Can you work these out from the model? Positions are in its coordinate system, mm. Coordinates: 2 decimals unless noted, no trailing zeros. Order: outer loops, then holes, each group sorted by start corner. A loop starts at its lowest first (then second) coordinate and runs counter-clockwise, first axis right, second up. Notation, with made-up numbers: (-32, -7.5) -> (-6, -7.5) arc R17 cw to (-6, 19.5) -> close; hole circle Ø5 at (64.5, -28). An arc over 180 degrees is marked (long way). Answer in a Markdown table with one row per item. Add a question column.
1. If I drill on line 1 along Z through (x, y) = (0, 12.95); line 2 along Y through (x, z) = (1, 5.5); line 3 along Z through (x, y) = (12.5, -8), over which ranges is the centre line in solid material (lowest first)? Write a range as [from, to].
2. Imagine slicing it at A-A on z = 31.5. Write out the boundary of the cut face in (x, y), plus the area to 3 significant figures.
3. Imagine slicing it at B-B on y = 0. Write out the boundary of the cut face in (x, z).
4. Imagine slicing it at C-C on x = -6. Write out the boundary of the cut face in (y, z), plus the area to 3 significant figures.
5. Will these pins go through, and if not, where does the flat tip stop? pin 1 (0.9 mm diameter, centred on y = 14, z = 34, fed in from -X); pin 2 (2 mm diameter, centred on x = 12.5, y = -1, fed in from +Z); pin 3 (3 mm diameter, centred on x = 7, z = 35, fed in from +Y); pin 4 (10 mm diameter, centred on x = 3.5, z = 16.5, fed in from +Y).
6. Imagine slicing it at D-D on z = 37.5. Write out the boundary of the cut face in (x, y), plus the area to 3 significant figures.
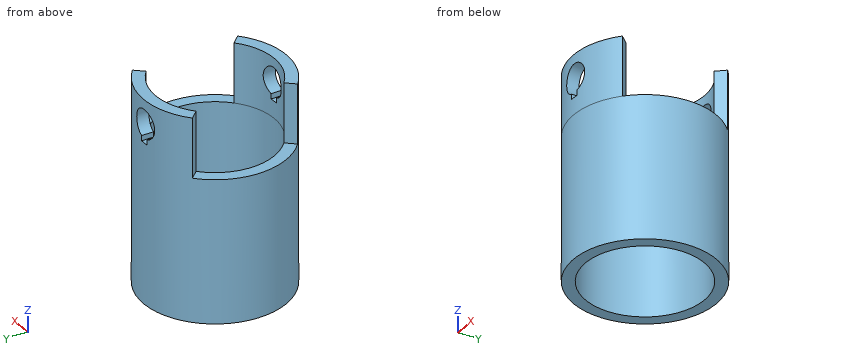
from build123d import *

# Parameters (mm, degrees)
SKETCH1_R           = 15
SKETCH1_R_2         = 12.5
BOSS_EXTRUDE1_DEPTH = 30
BOSS_EXTRUDE2_DEPTH = 12.5
CUT_EXTRUDE1_DEPTH  = 35


with BuildPart() as part:
    # Sketch1 → Boss-Extrude1 (new body)
    with BuildSketch(Plane(origin=(0, 0, 0), x_dir=(0, 1, 0), z_dir=(0, 0, 1))):
        Circle(SKETCH1_R)
        Circle(SKETCH1_R_2, mode=Mode.SUBTRACT)
    extrude(amount=BOSS_EXTRUDE1_DEPTH)

    # Sketch4 → Boss-Extrude2 (add)
    with BuildSketch(Plane.XY.offset(30)):
        with BuildLine():
            Line((-10, -11.180339887), (-8.333333333, -9.316949906))
            ThreePointArc((-8.333333333, -9.316949906), (0, -12.5), (8.333333333, -9.316949906))
            Line((8.333333333, -9.316949906), (10, -11.180339887))
            ThreePointArc((10, -11.180339887), (0, -15), (-10, -11.180339887))
        make_face()
        with BuildLine():
            Line((-10, 11.180339887), (-8.333333333, 9.316949906))
            ThreePointArc((-8.333333333, 9.316949906), (0, 12.5), (8.333333333, 9.316949906))
            Line((8.333333333, 9.316949906), (10, 11.180339887))
            ThreePointArc((10, 11.180339887), (0, 15), (-10, 11.180339887))
        make_face()
    extrude(amount=BOSS_EXTRUDE2_DEPTH)

    # Sketch6 → Cut-Extrude1 (cut)
    with BuildSketch(Plane(origin=(0, 15, 0), x_dir=(1, 0, 0), z_dir=(0, 1, 0))):
        with BuildLine():
            Line((-0.9, -34.638182396), (-0.9, -33.538182396))
            Line((-0.9, -33.538182396), (0.9, -33.538182396))
            Line((0.9, -33.538182396), (0.9, -34.638182396))
            ThreePointArc((0.9, -34.638182396), (0, -40.5), (-0.9, -34.638182396))
        make_face()
    extrude(amount=-CUT_EXTRUDE1_DEPTH, mode=Mode.SUBTRACT)


solid = part.part
Answers follow:
| question | item | result |
|---|---|---|
| 1 | line 1 | z = [0, 33.54], [40.5, 42.5] |
| 1 | line 2 | y = [-14.97, -12.46], [12.46, 14.97] |
| 1 | line 3 | z = [0, 30] |
| 2 | outline | (-10, -11.18) arc R15 ccw to (10, -11.18) -> (8.33, -9.32) arc R12.5 cw to (-8.33, -9.32) -> close; (-10, 11.18) -> (-8.33, 9.32) arc R12.5 cw to (8.33, 9.32) -> (10, 11.18) arc R15 ccw to start |
| 2 | area | 100 mm² |
| 3 | outline | (-15, 0) -> (-12.5, 0) -> (-12.5, 30) -> (-15, 30) -> close; (12.5, 0) -> (15, 0) -> (15, 30) -> (12.5, 30) -> close |
| 4 | outline | (-13.75, 0) -> (-10.97, 0) -> (-10.97, 42.5) -> (-13.75, 42.5) -> close; (10.97, 0) -> (13.75, 0) -> (13.75, 42.5) -> (10.97, 42.5) -> close |
| 4 | area | 236 mm² |
| 5 | pin 1 | stops at x = -6.43 |
| 5 | pin 2 | stops at z = 30 |
| 5 | pin 3 | stops at y = 13.96 |
| 5 | pin 4 | stops at y = 15 |
| 6 | outline | (-10, -11.18) arc R15 ccw to (-3, -14.7) -> (-3, -12.13) arc R12.5 cw to (-8.33, -9.32) -> close; (-10, 11.18) -> (-8.33, 9.32) arc R12.5 cw to (-3, 12.13) -> (-3, 14.7) arc R15 ccw to start; (3, -14.7) arc R15 ccw to (10, -11.18) -> (8.33, -9.32) arc R12.5 cw to (3, -12.13) -> close; (3, 12.13) arc R12.5 cw to (8.33, 9.32) -> (10, 11.18) arc R15 ccw to (3, 14.7) -> close |
| 6 | area | 70.1 mm² |
